Input: part model. Units: mm. Frame: model coordinates. Face numbers are marked on the shaded views. Give positions to 0.01 mm unless a question says otherwise; leave off trailing zeros. Write each loop counter-clockwise with the first axis right and the second up, starting at its lowest first coordinate (ties: lowest second). Pieces come first, ordered by that corner, then holes. Notation, with made-up numbers: (-24.5, 61) - (-13.5, 61) arc R17 cw to (-13.5, 74) - close; hole circle Ø9 at (-39.5, 11.25). An arc over 180 degrees is marked (long way). Use a Markdown table: item, result. Add a question column.
1. Section query C-C, the plane z = 33. Return loops of the section in (x, y).
2. Section query A-A, the plane y = 2.05. Return loops of the section in (x, z), plus the area to 3 significant figures.
3. Material intervals for probe 1 along X at (y, z) = (2.5, 18); probe 2 along X at (y, z) = (2.7, 25); probe 3 along Z at (x, y) = (-10.5, 1.8), sorted ascending.
4. Pin query (flat end, axial travel): pin 1 (18.5 mm diameter, centred on x = -7, z = 6.5, fed in from +Y). Return the tip coordinate at first contact, or that it passes through.
5. Mould query, pull axis Z, two halves, no side actions, for the marked faces 1 and 2. Classes: released by +Z, released by -Z, zero draft, split by the parting line, or undercut.
6. Section query D-D, the plane z = 26. Return loops of the section in (x, y).
7. Section query B-B, the plane x = -16.5. Return loops of the section in (y, z).
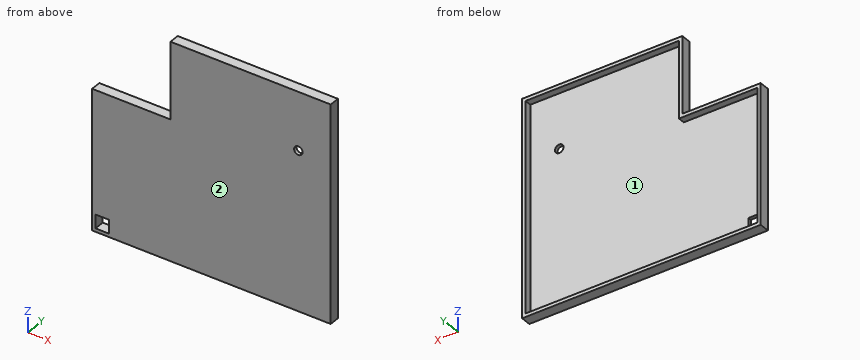
```python
from build123d import *

# Parameters (mm, degrees)
BOSS_EXTRUDE1_DEPTH = 3
CUT_EXTRUDE2_START  = 1
CUT_EXTRUDE2_DEPTH  = 55.91287866
SKETCH2_R           = 1.25
CUT_EXTRUDE3_DEPTH  = 56.868148349
CUT_EXTRUDE4_REACH  = 57.868
SKETCH3_W           = 4
SKETCH3_H           = 4


with BuildPart() as part:
    # Sketch1 → Boss-Extrude1 (new body)
    # profile 1 of 2: a face of its own
    with BuildSketch(Plane(origin=(0, 0, 0), x_dir=(1, 0, 0), z_dir=(0, 1, 0))):
        Polygon((35, -18), (35, -20), (35, -43.5), (-12, -43.5), (-12, -21), (-35, -21), (-35, -18), (-35, 20), (35, 20), align=None)
        Polygon((34, -18), (34, 19), (-34, 19), (-34, -18), (-34, -20), (-11, -20), (-11, -42.5), (34, -42.5), (34, -20), align=None, mode=Mode.SUBTRACT)
    # profile 2 of 2: a face of its own
    with BuildSketch(Plane(origin=(0, 0, 0), x_dir=(1, 0, 0), z_dir=(0, 1, 0))):
        Polygon((34, -18), (34, -20), (34, -42.5), (-11, -42.5), (-11, -20), (-34, -20), (-34, -18), (-34, 19), (34, 19), align=None)
    extrude(amount=BOSS_EXTRUDE1_DEPTH)

    # Sketch1_6 → Cut-Extrude2 (cut, through all)
    with BuildSketch(Plane(origin=(0, 0, 0), x_dir=(1, 0, 0), z_dir=(0, 1, 0)).offset(CUT_EXTRUDE2_START)):
        Polygon((34, -18), (34, -20), (34, -42.5), (-11, -42.5), (-11, -20), (-34, -20), (-34, -18), (-34, 19), (34, 19), align=None)
    extrude(amount=CUT_EXTRUDE2_DEPTH, mode=Mode.SUBTRACT)

    # Sketch2 → Cut-Extrude3 (cut, through all)
    with BuildSketch(Plane(origin=(0, 1, 0), x_dir=(1, 0, 0), z_dir=(0, 1, 0))):
        with Locations(Location((25.514070345, -26.486113073, 0), (0, 0, 270))):
            Circle(SKETCH2_R)
    extrude(amount=-CUT_EXTRUDE3_DEPTH, mode=Mode.SUBTRACT)

    # Sketch3 → Cut-Extrude4 (cut, up to next)
    with BuildSketch(Plane(origin=(0, 1, 0), x_dir=(1, 0, 0), z_dir=(0, 1, 0)), mode=Mode.PRIVATE) as cut_extrude4_sk1:
        with Locations((-32, 17)):
            Rectangle(SKETCH3_W, SKETCH3_H)
    cut_extrude4_tool1 = extrude(cut_extrude4_sk1.sketch, amount=-CUT_EXTRUDE4_REACH, mode=Mode.PRIVATE) & part.part
    add(cut_extrude4_tool1.solids().sort_by_distance((-32, 1, -17))[0], mode=Mode.SUBTRACT)


solid = part.part
```
Result sheet:
| question | item | result |
|---|---|---|
| 1 | outline | (-12, 0) - (35, 0) - (35, 3) - (34, 3) - (34, 1) - (-11, 1) - (-11, 3) - (-12, 3) - close |
| 2 | outline | (-35, -20) - (35, -20) - (35, 43.5) - (-12, 43.5) - (-12, 21) - (-35, 21) - close; hole (-34, -19) - (34, -19) - (34, 42.5) - (-11, 42.5) - (-11, 20) - (-34, 20) - close |
| 2 | area | 263 mm² |
| 3 | probe 1 | x = -35 to -34, 34 to 35 |
| 3 | probe 2 | x = -12 to -11, 34 to 35 |
| 3 | probe 3 | z = -20 to -19, 42.5 to 43.5 |
| 4 | pin 1 | stops at y = 1 |
| 5 | face 1 | undercut |
| 5 | face 2 | zero draft |
| 6 | outline | (-12, 0) - (24.36, 0) - (24.36, 1) - (-11, 1) - (-11, 3) - (-12, 3) - close; (26.67, 0) - (35, 0) - (35, 3) - (34, 3) - (34, 1) - (26.67, 1) - close |
| 7 | outline | (0, -20) - (3, -20) - (3, -19) - (1, -19) - (1, 20) - (3, 20) - (3, 21) - (0, 21) - close |
